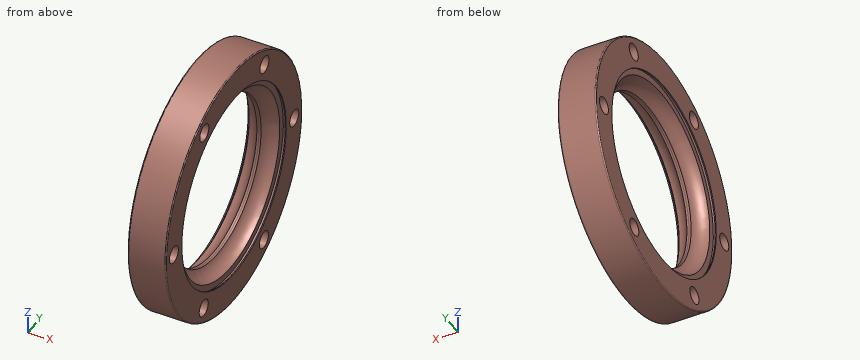
```python
from build123d import *

# Parameters (mm, degrees)
F2_R     = 0.5
F4_R     = 4
F5_DEPTH = 18


with BuildPart() as f1:
    # F0 (on Front) → F1 (revolve)
    with BuildSketch(Plane.XZ):
        with BuildLine():
            Line((9, 60), (0, 60))
            Line((0, 60), (0, 38.75))
            Line((0, 38.75), (1, 38.75))
            ThreePointArc((1, 38.75), (3.422249, 42.041403), (7.2, 43.6))
            Line((7.2, 43.6), (7.2, 46))
            Line((7.2, 46), (7.2, 46.751757))
            Line((7.2, 46.751757), (8.5, 46.751757))
            Line((8.5, 46.751757), (8.5, 46))
            Line((8.5, 46), (9, 46))
            Line((9, 46), (9, 60))
        make_face()
    revolve(axis=Axis((13.202514, 0, 0), (1, 0, 0)))

    # F2
    f2_edges = [f1.edges().sort_by_distance(p)[0] for p in [
        (9, 0, -60),
    ]]
    fillet(f2_edges, radius=F2_R)

    # F3: F1 across face


with BuildPart() as f1_1:
    add(f1.part)
    add(f1.part.mirror(Plane(origin=(0, 0, 0), x_dir=(0, -1, 0), z_dir=(-1, 0, 0))))

    # F4 (on face) → F5 (cut)
    with BuildSketch(Plane.YZ.offset(9)):
        with Locations((-52.995591, 0.275232)):
            Circle(F4_R)
        with Locations((-26.217681, 46.06119)):
            Circle(F4_R)
        with Locations((26.736153, 45.757913)):
            Circle(F4_R)
        with Locations((52.995591, -0.275232)):
            Circle(F4_R)
        with Locations((26.261273, -46.036364)):
            Circle(F4_R)
        with Locations((-26.736153, -45.757913)):
            Circle(F4_R)
    extrude(amount=-F5_DEPTH, mode=Mode.SUBTRACT)


solid = f1_1.part
```
Here's how the part is built. I have some questions about the finished solid (model axes, mm). Coordinates: 2 decimals unless noted, no trailing zeros. Order: outer loops, then holes, each group sorted by start corner. A loop starts at its lowest first (then second) coordinate and runs counter-clockwise, first axis right, second up.
Item 1: I need wall thicknesses on probe 1 along Z at (x, y) = (7.95, 0); probe 2 along Y at (x, z) = (-0.4, 0); probe 3 along Z at (x, y) = (5.5, -29.5). Which ranges of each line are inside material? Lowest first, please.
Response values:
probe 1: z = -60 to -46.75, 46.75 to 60
probe 2: y = -60 to -56.99, -49.01 to -38.75, 38.75 to 49.01, 56.99 to 60
probe 3: z = -52.25 to -48.65, -42.87 to -31.55, 31.55 to 43.78, 48.35 to 52.25
Item 2: If we section it at B-B, the plane x = 5.75: List the corners of the cut face in (y, z) for me.
Response values:
outline: circle Ø120 at (0, 0); hole circle Ø8 at (-53, 0.28); hole circle Ø86.56 at (0, 0); hole circle Ø8 at (-26.74, -45.76); hole circle Ø8 at (-26.22, 46.06); hole circle Ø8 at (26.26, -46.04); hole circle Ø8 at (26.74, 45.76); hole circle Ø8 at (53, -0.28)
Item 3: If we section it at C-C, the plane x = -3.75: List the corners of the cut face in (y, z) for me.
Response values:
outline: circle Ø120 at (0, 0); hole circle Ø8 at (-53, 0.28); hole circle Ø84.57 at (0, 0); hole circle Ø8 at (-26.74, -45.76); hole circle Ø8 at (-26.22, 46.06); hole circle Ø8 at (26.26, -46.04); hole circle Ø8 at (26.74, 45.76); hole circle Ø8 at (53, -0.28)
Item 4: I'm going to push flat-ended pins straight in: pin 1 Ø6 at (x, z) = (3.5, 5) entering from +Y; pin 2 Ø9 at (y, z) = (-53, 0.28) entering from +X; pin 3 Ø4 at (x, y) = (-3.5, -13) entering from -Z; pin 4 Ø5 at (y, z) = (26.74, 45.76) entering from -X. Where does each tip first touch, or does it pass through?
Response values:
pin 1: stops at y = 59.97
pin 2: stops at x = 9
pin 3: stops at z = -58.98
pin 4: passes through
